The figure shows three views and two pictorial views of one solid part (mm, origin at its lowest corner). Answer the questions. A direction names the side the tool comes from. Round coordinates to 2 decimals unless told otherwise and drop trailing zeros. Write each loop counter-clockwise with the first axis right and the second up, starting at its lowest first coordinate (ties: lowest second). Pieces come first, ordered by that corner, then holes.
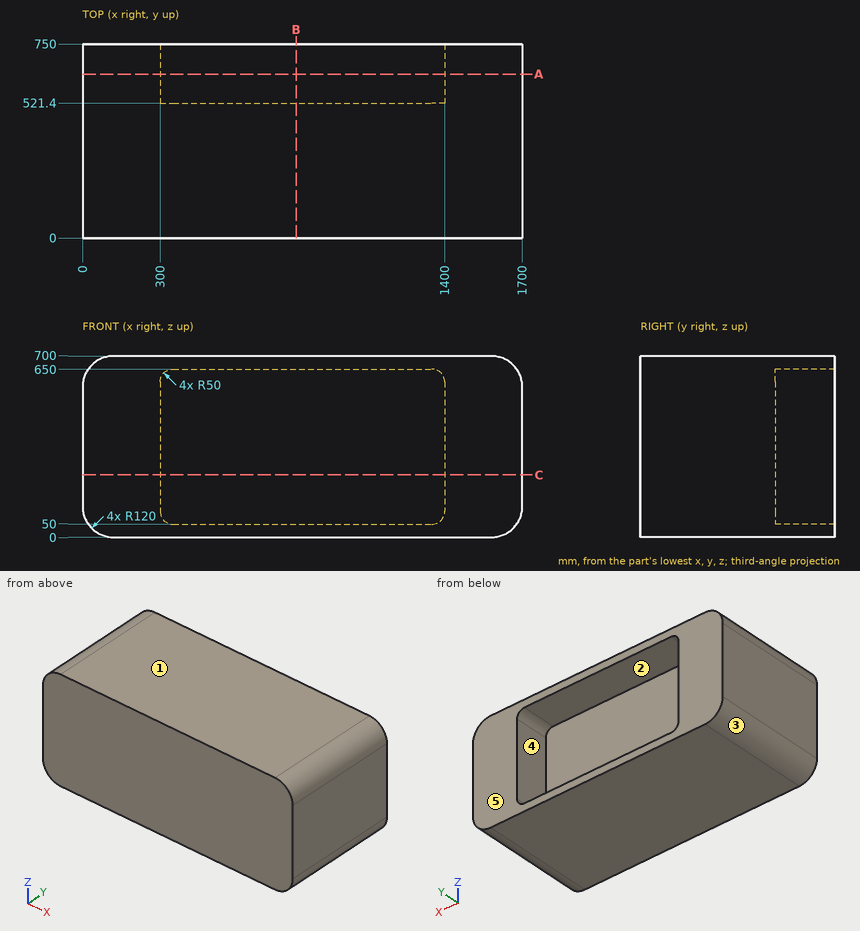
Q1. Section C-C (z = 241) is taken. Determine the outline of the cut face in (x, y).
Verdict:
outline: (0, 0) - (1700, 0) - (1700, 750) - (1400, 750) - (1400, 521.4) - (300, 521.4) - (300, 750) - (0, 750) - close
Q2. Flat-ended cylindrical pins translate along their axes: pin 1 Ø3 at (y, z) = (591.5, 354) entering from -X; pin 2 Ø1.5 at (x, z) = (328.5, 120) entering from +Y. Find the tip coordinate at first contact, or state that the pin passes through.
Verdict:
pin 1: stops at x = 0
pin 2: stops at y = 521.4
Q3. Section A-A (y = 633.5) is taken. Determine the outline of the cut face in (x, z), then the cut area to 3 significant figures.
Verdict:
outline: (0, 120) arc R120 ccw to (120, 0) - (1580, 0) arc R120 ccw to (1700, 120) - (1700, 580) arc R120 ccw to (1580, 700) - (120, 700) arc R120 ccw to (0, 580) - close; hole (300, 100) arc R50 ccw to (350, 50) - (1350, 50) arc R50 ccw to (1400, 100) - (1400, 600) arc R50 ccw to (1350, 650) - (350, 650) arc R50 ccw to (300, 600) - close
area: 520,000 mm2
Q4. Which of the six approach directions +Z, -Z, +X, -X, +Y, -Y give full straight-line access (tool end or side, diameter ignored) to the marked faces 4 and 5?
Verdict:
face 4: +Y
face 5: +Z, -Z, +X, -X, +Y
Q5. Determine the mould class of the marked faces 1, 2 and 3 for opening direction Z: pulls with the +Z half, pulls with the -Z half, needs draft (parallel to the pull), parting line crosses it, or undercut.
Verdict:
face 1: pulls with the +Z half
face 2: undercut
face 3: pulls with the -Z half
Q6. Straight lines are drawn through the part: probe 1 along X at (y, z) = (537.5, 162); probe 2 along X at (y, z) = (271, 117); probe 3 along Y at (x, z) = (895.5, 314.5). For each, find the intervals that lie inside material, in ascending order.
Verdict:
probe 1: x = 0 to 300, 1400 to 1700
probe 2: x = 0.04 to 1699.96
probe 3: y = 0 to 521.4
Q7. Section B-B (x = 825.5) is taken. Determine the outline of the cut face in (y, z), then the cut area to 3 significant figures.
Verdict:
outline: (0, 0) - (750, 0) - (750, 50) - (521.4, 50) - (521.4, 650) - (750, 650) - (750, 700) - (0, 700) - close
area: 388,000 mm2
